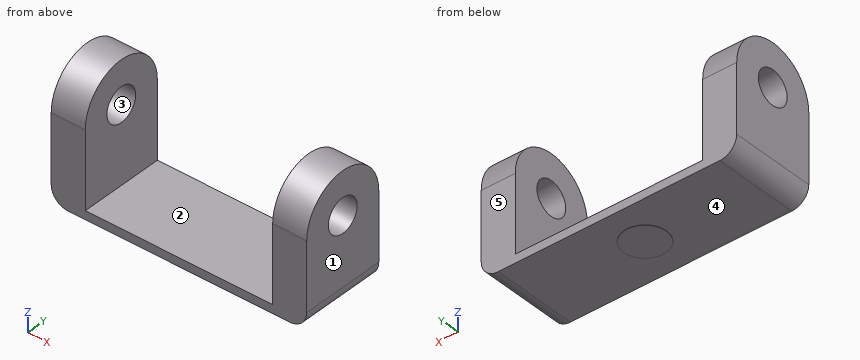
Autodesk Inventor part; units mm, degrees
ref_plane "YZ Plane" through (0, 0, 0) normal (1, 0, 0) x (0, 1, 0)
ref_plane "XZ Plane" through (0, 0, 0) normal (0, 1, 0) x (-1, 0, 0)
ref_plane "XY Plane" through (0, 0, 0) normal (0, 0, 1) x (1, 0, 0)
sketch "Sketch1" plane through (0, 0, 0) normal (0, 0, 1) x (1, 0, 0)
  line L0 (0, 0) -> (30, 0)
  line L1 (30, -20) -> (0, -20)
  line L2 (0, 0) -> (0, -20)
  line L3 (0, 0) -> (-30, 0)
  line L4 (-30, -20) -> (0, -20)
  line L5 (30, 0) -> (30, -20)
  line L6 (-30, 0) -> (-30, -20)
  dimension "d0" = 30
  dimension "d6" = 20
extrude "Extrusion1" add sketch "Sketch1" along normal mid plane 2
sketch "Sketch2" plane through (-28, -20, -1) normal (-1, 0, 0) x (0, -1, 0)
  line L0 (-20, 0) -> (0, 0)
  line L1 (0, 0) -> (0, 30)
  line L2 (0, 30) -> (-20, 30)
  line L3 (-20, 30) -> (-20, 0)
edge flange "Flange1" height 30 angle 90 thickness 2 bend radius 2 thickness toward (-1, 0, 0) relief tear relief width 2 relief depth 1 edges at (-30, -10, 1) wall of the first edge with corners at (-28, 0, -1) (-28, -20, -1) (-28, -20, 29) (-28, 0, 29)
bend "Bend1"
corner "Corner1"
sketch "Sketch3" plane through (28, 0, -1) normal (1, 0, 0) x (0, 1, 0)
  line L0 (-20, 0) -> (0, 0)
  line L1 (0, 0) -> (0, 30)
  line L2 (0, 30) -> (-20, 30)
  line L3 (-20, 30) -> (-20, 0)
edge flange "Flange2" height 30 angle 90 thickness 2 bend radius 2 thickness toward (1, 0, 0) relief tear relief width 2 relief depth 1 edges at (30, -10, 1) wall of the first edge with corners at (28, -20, -1) (28, 0, -1) (28, 0, 29) (28, -20, 29)
bend "Bend2"
corner "Corner2"
sketch "Sketch5" plane through (30, -20, 29) normal (1, 0, 0) x (0, 0, -1)
  line L0 (26, 0) -> (0, 0)
  line L1 (0, 0) -> (0, 20)
  line L2 (0, 20) -> (0, 0)
  line L3 (0, 0) -> (0, 20)
  line L4 (0, 20) -> (10, 20)
  line L5 (0, 0) -> (10, 0)
  line L6 (0, 0) -> (26, 0)
  arc A0 (10, 20) -> (10, 0) centre (10, 10) ccw
  line L7 (0, 20) -> (26, 20)
  circle A1 centre (10, 10) radius 4
  point P0 (29, 20)
  point P1 (0, 10)
  dimension "d38" = 10
  dimension "d39" = 10
  dimension "d40" = 10
  dimension "d46" = 8
extrude "Cut1" cut sketch "Sketch5" against normal blind 2
sketch "Sketch6" plane through (-30, -20, 29) normal (-1, 0, 0) x (0, 0, 1)
  line L0 (0, 20) -> (0, 0)
  line L1 (-10, 0) -> (0, 0)
  line L2 (0, 0) -> (0, 20)
  line L3 (0, 20) -> (-10, 20)
  line L4 (-26, 20) -> (0, 20)
  arc A0 (-10, 0) -> (-10, 20) centre (-10, 10) ccw
  circle A1 centre (-10, 10) radius 4
  point P0 (-29, 20)
  point P1 (0, 10)
  dimension "d43" = 10
  dimension "d47" = 8
extrude "Cut2" cut sketch "Sketch6" against normal blind 2
sketch "Sketch8" plane through (-30, -20, 3) normal (-1, 0, 0) x (0, 0, 1)
  line L0 (16, 0) -> (0, 0)
  arc A0 (16, 0) -> (16, 20) centre (16, 10) ccw
  line L1 (0, 20) -> (16, 20)
  line L2 (0, 20) -> (0, 0)
  line L3 (16, 0) -> (0, 0)
  arc A1 (16, 0) -> (16, 20) centre (16, 10) ccw
  line L4 (0, 0) -> (16, 0)
  arc A2 (16, 0) -> (16, 20) centre (16, 10) ccw
  line L5 (16, 20) -> (0, 20)
  line L6 (16, 20) -> (0, 20)
  line L7 (0, 20) -> (0, 0)
  line L8 (0, 20) -> (0, 0)
  circle A3 centre (16, 10) radius 4
  point P0 (-3, 20)
extrude "Extrusion3" add sketch "Sketch8" against normal blind 8
sketch "Sketch9" plane through (28, -20, 3) normal (-1, 0, 0) x (0, 0, 1)
  line L0 (0, 0) -> (16, 0)
  line L1 (0, 0) -> (16, 0)
  line L2 (16, 0) -> (0, 0)
  arc A0 (16, 0) -> (16, 20) centre (16, 10) ccw
  arc A1 (16, 0) -> (16, 20) centre (16, 10) ccw
  line L3 (0, 0) -> (0, 20)
  line L4 (16, 20) -> (0, 20)
  line L5 (0, 20) -> (0, 0)
  circle A2 centre (16, 10) radius 4
  circle A3 centre (16, 10) radius 4
  point P0 (-3, 20)
extrude "Extrusion4" add sketch "Sketch9" along normal blind 6
sketch "Sketch11" plane through (-22, 0, 3) normal (0, 0, -1) x (-1, 0, 0)
  line L0 (6, 0) -> (0, 0)
  line L1 (0, 0) -> (6, 0)
  line L2 (6, -20) -> (6, 0)
  line L3 (6, 0) -> (6, -20)
  line L4 (6, -20) -> (0, -20)
  line L5 (6, -20) -> (0, -20)
  line L6 (0, 0) -> (0, -20)
  line L7 (0, -20) -> (0, 0)
  point P0 (-22, 0)
extrude "Extrusion5" add sketch "Sketch11" along normal blind 3
sketch "Sketch12" plane through (28, -20, 3) normal (0, 0, -1) x (-1, 0, 0)
  line L0 (2, 20) -> (0, 20)
  line L1 (6, 20) -> (6, 0)
  line L2 (0, 20) -> (6, 20)
  line L3 (6, 20) -> (6, 0)
  line L4 (2, 0) -> (0, 0)
  line L5 (6, 0) -> (0, 0)
  line L6 (0, 20) -> (0, 0)
  line L7 (0, 0) -> (0, 20)
  point P0 (28, 20)
extrude "Extrusion6" add sketch "Sketch12" along normal blind 3
sketch "Sketch13" plane through (0, 0, -1) normal (0, 0, -1) x (-1, 0, 0)
  circle A0 centre (0, -10) radius 5
  line L0 (26, -20) -> (26, 0)
  point P0 (0, 0)
  dimension "d62" = 10
  dimension "d63" = 10
  dimension "d64" = 26
extrude "Extrusion7" add sketch "Sketch13" along normal blind 0.1
equation "\"d41\" = Thickness"
equation "\"d44\" = Thickness"
equation "\"d7\" = Thickness"
equation "\"d8\" = BendReliefWidth"
equation "\"d9\" = BendReliefDepth"
equation "\"d10\" = MinimumRemnant"
equation "\"d11\" = TransitionRadius"
equation "\"d14\" = BendRadius"
equation "\"d15\" = CornerReliefSize"
equation "\"d16\" = GapSize"
equation "\"d17\" = JacobiRadiusSize"
equation "\"d18\" = BendReliefWidth"
equation "\"d19\" = BendReliefDepth"
equation "\"d20\" = MinimumRemnant"
equation "\"d21\" = TransitionRadius"
equation "\"d24\" = BendRadius"
equation "\"d25\" = CornerReliefSize"
equation "\"d26\" = GapSize"
equation "\"d27\" = JacobiRadiusSize"
equation "\"BendRadius\" = Thickness"
equation "\"BendReliefWidth\" = Thickness"
equation "\"BendReliefDepth\" = 0.5 * Thickness"
equation "\"CornerReliefSize\" = 4 * Thickness"
equation "\"MinimumRemnant\" = 2 * Thickness"
equation "\"TransitionRadius\" = BendRadius"
equation "\"JacobiRadiusSize\" = BendRadius"
equation "\"GapSize\" = Thickness"
properties part number "SHEET_METAL1"
Could you check a few things on this model? Use its own coordinates, in mm. Face numbers are marked on the shaded views. A direction names the side the tool comes from. Round coordinates to 2 decimals unless told otherwise and drop trailing zeros. Loops run counter-clockwise (first coordinate to the right, second up) from the corner with the lowest first, then second, coordinate; pieces in that order, holes last. Notation, with made-up numbers: (24.25, 78) -> (43.25, 78) arc R25 cw to (43.25, 102) -> close; hole circle Ø7 at (54, 15.25). An arc over 180 degrees is marked (long way). Put each result on its own line as item: value.
Q1. I want a section at B-B on y = -10. Write out the boundary of the cut face in (x, z), and give its area (3 significant figures).
Checks:
outline: (-30, 3) arc R4 ccw to (-26, -1) -> (-5, -1) -> (-5, -1.1) -> (5, -1.1) -> (5, -1) -> (26, -1) arc R4 ccw to (30, 3) -> (30, 15) -> (22, 15) -> (22, 1) -> (-22, 1) -> (-22, 15) -> (-30, 15) -> close; (-30, 23) -> (-22, 23) -> (-22, 29) -> (-30, 29) -> close; (22, 23) -> (30, 23) -> (30, 29) -> (22, 29) -> close
area: 434 mm2
Q2. Which directions (+Z, -Z, +X, -X, +Y, -Y) give clear straight access to the entire face, cutting with the end or side of a thin tool? Please do the marked faces 1 and 2.
Checks:
face 1: +Z, -Z, +X, +Y, -Y
face 2: +Z, +Y, -Y
Q3. For pin 1 Ø3 at (x, y) = (8.5, -10.5) entering from -Z; pin 2 Ø4 at (x, y) = (-2, -14.5) entering from +Z; pin 3 Ø7 at (y, z) = (-10, 19) entering from -X, each with a flat end and sliding along its axis, tell me the tip position at first contact or that it passes through.
Checks:
pin 1: z = -1
pin 2: z = 1
pin 3: through
Q4. Thinking about a two-plate mould opening in Y: for the marked faces 3, 4 and 5, which applies, pulls with the +Y half, pulls with the -Y half, needs draft (parallel to the pull), parting line crosses it, or undercut?
Checks:
face 3: undercut
face 4: needs draft
face 5: pulls with the +Y half
Q5. I want a section at D-D on x = 0. Write out the boundary of the cut face in (y, z), and give its area (3 significant figures).
Checks:
outline: (-20, -1) -> (-15, -1) -> (-15, -1.1) -> (-5, -1.1) -> (-5, -1) -> (0, -1) -> (0, 1) -> (-20, 1) -> close
area: 41.0 mm2
Q6. I want a section at A-A on z = 12.5. Write out the boundary of the cut face in (x, y), and give its area (3 significant figures).
Checks:
outline: (-30, -20) -> (-22, -20) -> (-22, 0) -> (-30, 0) -> close; (22, -20) -> (30, -20) -> (30, 0) -> (22, 0) -> close
area: 320 mm2
Q7. Please list where these lines run through material, in increasing order: line 1 (X direction, y = -11, z = 11); line 2 (Y direction, x = 24.75, z = 19); line 3 (Z direction, x = 24.5, y = -10). Write a range as from..to.
Checks:
line 1: -30..-22, 22..30
line 2: -20..-14, -6..0
line 3: -1..15, 23..29
Q8. I want a section at C-C on x = -23. Write out the boundary of the cut face in (y, z).
Checks:
outline: (-20, -1) -> (0, -1) -> (0, 19) arc R10 ccw to (-20, 19) -> close; hole circle Ø8 at (-10, 19)
